CAD build for the part. Positions are in the model's coordinates, mm. Round coordinates to 2 decimals unless told otherwise and drop trailing zeros. Order: outer loops, then holes, each group sorted by start corner. A loop starts at its lowest first (then second) coordinate and runs counter-clockwise, first axis right, second up. Notation, with made-up numbers: M 76.25,67 L 99.25,67 A17 cw 99.25,81 Z; hole C -1,35.5 d5. An arc over 180 degrees is marked long. Put each result on its own line as item: value.
Autodesk Inventor part; units mm, degrees
ref_plane "YZ Plane" through (0, 0, 0) normal (1, 0, 0) x (0, 1, 0)
ref_plane "XZ Plane" through (0, 0, 0) normal (0, 1, 0) x (-1, 0, 0)
ref_plane "XY Plane" through (0, 0, 0) normal (0, 0, 1) x (1, 0, 0)
sketch "Эскиз1" plane through (0, 0, 0) normal (0, 1, 0) x (-1, 0, 0)
  line L0 (18, -16) -> (-18, -16)
  line L1 (-18, -16) -> (-18, 16)
  line L2 (-18, 16) -> (18, 16)
  line L3 (18, 16) -> (18, -16)
  line L4 (14.82, -12.82) -> (-14.82, -12.82)
  line L5 (-14.82, -12.82) -> (-14.82, 12.82)
  line L6 (-14.82, 12.82) -> (14.82, 12.82)
  line L7 (14.82, 12.82) -> (14.82, -12.82)
  circle A0 centre (14.82, -12.82) radius 1.5
  circle A1 centre (14.82, 12.82) radius 1.5
  circle A2 centre (-14.82, 12.82) radius 1.5
  circle A3 centre (-14.82, -12.82) radius 1.5
  arc A4 (11.9634, -10.02) -> (14.12, -8.8817) centre (14.82, -12.82) ccw
  circle A5 centre (-14.82, -12.82) radius 4
  arc A6 (14.12, 8.8817) -> (12.7129, 9.42) centre (14.82, 12.82) ccw
  arc A7 (-11.0303, 14.1) -> (-16.6, 9.2379) centre (-14.82, 12.82) ccw
  line L8 (14.12, -10.02) -> (1.12, -10.02)
  line L9 (1.12, -10.02) -> (1.12, 9.42)
  line L10 (1.12, 9.42) -> (14.12, 9.42)
  line L11 (14.12, 9.42) -> (14.12, -10.02)
  line L12 (-9.6, 7.9) -> (-16.6, 7.9)
  line L13 (-16.6, 7.9) -> (-16.6, 14.1)
  line L14 (-16.6, 14.1) -> (-9.6, 14.1)
  line L15 (-9.6, 14.1) -> (-9.6, 7.9)
  line L16 (-11.0303, 14.1) -> (-16.6, 14.1)
  line L17 (14.12, 8.8817) -> (14.12, 9.42)
  line L18 (14.12, -8.8817) -> (14.12, -10.02)
  line L19 (11.9634, -10.02) -> (14.12, -10.02)
  circle A8 centre (-13.034, 10.913) radius 1.5
  circle A9 centre (-13.034, 10.913) radius 1.25
  line L20 (20, -18) -> (-20, -18)
  line L21 (-20, -18) -> (-20, 18)
  line L22 (-20, 18) -> (20, 18)
  line L23 (20, 18) -> (20, -18)
  line L24 (-10.82, -12.82) -> (-10.82, -16)
  line L25 (-14.82, -8.82) -> (-18, -8.82)
  line L26 (10.82, -12.82) -> (10.82, -16)
  line L27 (14.82, -8.82) -> (18, -8.82)
  line L28 (14.82, 8.82) -> (18, 8.82)
  line L29 (10.82, 12.82) -> (10.82, 16)
  line L30 (-18, 8.82) -> (-16.6, 8.82)
  line L31 (-10.82, 16) -> (-10.82, 14.1)
  line L32 (-10.82, 14.1) -> (-11.0303, 14.1)
  line L33 (-16.6, 9.2379) -> (-16.6, 8.82)
  line L34 (3.5, 16) -> (3.5, 12.6)
  line L35 (3.5, 12.6) -> (-8.2, 12.6)
  line L36 (-8.2, 12.6) -> (-8.2, 16)
  line L37 (-6.7, 18) -> (-6.7, 13.6)
  line L38 (-6.7, 13.6) -> (2, 13.6)
  line L39 (2, 13.6) -> (2, 18)
  line L40 (3.5, 16) -> (3.5, 12.6)
  line L41 (-8.2, 12.6) -> (3.5, 12.6)
  line L42 (-8.2, 12.6) -> (-8.2, 16)
  line L43 (-8.2, 16) -> (-6.7, 16)
  line L44 (-6.7, 16) -> (-6.7, 13.6)
  line L45 (-6.7, 13.6) -> (2, 13.6)
  line L46 (2, 13.6) -> (2, 16)
  line L47 (2, 16) -> (3.5, 16)
  line L48 (-10.82, 14.1) -> (-8.2, 14.1)
  line L49 (-8.2, 14.1) -> (-8.2, 16)
  line L50 (3.5, 12.6) -> (10.8261, 12.6)
  line L51 (10.8261, 12.6) -> (10.82, 12.82)
  line L52 (10.82, 12.82) -> (3.5, 12.82)
  line L53 (3.5, 12.82) -> (3.5, 12.6)
  line L54 (-16.6, 7.9) -> (-16.6, -8.82)
  line L55 (-16.6, -8.82) -> (-18, -8.82)
  line L56 (-18, -8.82) -> (-18, 8.82)
  point P0 (0, 0)
  dimension "d0" = 36
  dimension "d1" = 32
  dimension "d2" = 3.18
  dimension "d3" = 3.18
  dimension "d4" = 3.18
  dimension "d5" = 3.18
  dimension "d6" = 3
  dimension "d7" = 3
  dimension "d8" = 3
  dimension "d9" = 3
  dimension "d10" = 8
  dimension "d11" = 8
  dimension "d12" = 8
  dimension "d13" = 8
  dimension "d14" = 2.8
  dimension "d15" = 0.7
  dimension "d16" = 3.4
  dimension "d17" = 13
  dimension "d18" = 1.9
  dimension "d19" = 1.4
  dimension "d20" = 7
  dimension "d21" = 6.2
  dimension "d22" = 4.966
  dimension "d23" = 5.087
  dimension "d24" = 3
  dimension "d25" = 2.5
  dimension "d26" = 2
  dimension "d27" = 2
  dimension "d28" = 2
  dimension "d29" = 2
  dimension "d30" = 4
  dimension "d31" = 4
  dimension "d32" = 16
  dimension "d33" = 11.3
  dimension "d34" = 1
  dimension "d35" = 1.5
  dimension "d36" = 1.5
  dimension "d37" = 2.4
extrude "Выдавливание1" add sketch "Эскиз1" along normal blind 1 contours L0 A4 L3 A6 L2 L39 L22 L23 L20 L21 L37 A7 L1 A5 | L26 A4 L0 | L0 L24 L4 L26 | L0 A5 L24 | A4 L4 A0 L7 L3 L0 | L0 A4 | A4 L8 L11 L7 A0 L4 | A5 L0 | L0 A5 L1 L5 A3 L4 | L4 A3 L5 A5 | A4 L3 L0 | A0 L7 L4 | L4 L7 A0 | L0 L1 A5 | A3 L5 L4 | L4 L5 A3 | A5 L1 L25 | L3 A4 | A5 L1 | A4 L27 L3 | L7 L28 L3 L27 | A6 L11 L10 L6 A1 L7 | L7 A1 L6 A6 L2 L3 | A6 L3 L28 | L14 L13 A7 L1 L2 A2 | A2 L14 | L30 L1 A7 L13 | A1 L6 L7 | L7 L6 A1 | L3 A6 | L36 L2 L37 L38 L39 L34 L6 | A7 L1 | A6 L2 L3 | L29 L2 A6 | A7 L2 L31 L14 | L1 L2 A7 | L2 A6 | L2 A7
extrude "Выдавливание2" add sketch "Эскиз1" along normal blind 1 contours L25 L1 L30 L13 L54 | L14 L13 A7 L1 L2 A2 | A2 L14 | L30 L1 A7 L13 | L50 L34 L6 A6 | L36 L2 L37 L38 L39 L34 L6 | L6 L34 L35 L36 | L14 L31 L2 L36 L48 | L6 L34 L2 L29 | A7 L2 L31 L14 | L1 L2 A7
extrude "Выдавливание3" cut sketch "Эскиз1" along normal blind 1 contours A0 L7 L4 | L4 L7 A0 | A3 L5 L4 | L4 L5 A3 | A1 L6 L7 | L7 L6 A1
equation "\"d6\" = d9"
equation "\"d7\" = d9"
equation "\"d8\" = d9"
properties part number "resin_top"
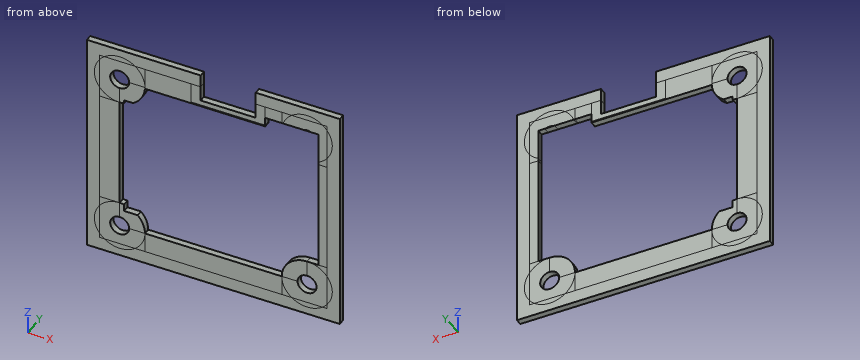
Item 1: Band-saw the part on B-B on z = 5. Give the cut face in (x, y).
Answers below:
outline: M -20,0 L -14.82,0 L -14.82,1 L -20,1 Z; M 16.6,0 L 20,0 L 20,1 L 16.6,1 Z
Item 2: Pin check, flat tips, straight feed: P1, Ø6, axis at x = 12, z = 11, coming from the -Y side; P2, Ø0.5, axis at x = 1, y = 0.5, coming from the +Z side. Stop position of each tip, or through.
Answers below:
P1: through
P2: z = 13.6
Item 3: Band-saw the part on C-C on y = 0.6. Give the cut face in (x, z).
Answers below:
outline: M -20,-18 L 20,-18 L 20,18 L 6.7,18 L 6.7,13.6 L -2,13.6 L -2,18 L -20,18 Z; hole C -14.82,-12.82 d3; hole C -14.82,12.82 d3; hole M -14.82,-8.82 A4 cw -14.12,-8.88 L -14.12,-10.02 L -11.96,-10.02 A4 cw -10.82,-12.82 L 10.82,-12.82 A4 cw 14.82,-8.82 L 16.6,-8.82 L 16.6,14.1 L 8.2,14.1 L 8.2,12.6 L -10.83,12.6 A4 cw -12.71,9.42 L -14.12,9.42 L -14.12,8.88 A4 cw -14.82,8.82 Z; hole C 14.82,-12.82 d3
Item 4: Band-saw the part on A-A on x = 10. Give the cut face in (y, z).
Answers below:
outline: M 0,-18 L 1,-18 L 1,-12.82 L 0,-12.82 Z; M 0,14.1 L 1,14.1 L 1,18 L 0,18 Z
Item 5: Probe line 1 along X through (y, z) = (0.1, 13); line 2 along Z through (x, y) = (14.82, 0.65); line 3 along X through (y, z) = (0.2, 15). List the from-to ranges inside material, lowest first. Write a range as [from, to].
Answers below:
line 1: [-20, -16.31], [-13.33, 8.2], [16.6, 20]
line 2: [-18, -14.32], [-11.32, -8.82], [14.1, 18]
line 3: [-20, -2], [6.7, 20]
